Read the model definition and answer for the solid it produces. Units are mm, in the model's axes. Coordinates: 2 decimals unless noted, no trailing zeros. Order: outer loops, then holes, each group sorted by start corner. A loop starts at its lowest first (then second) coordinate and runs counter-clockwise, first axis right, second up. Notation, with made-up numbers: (24, 71.25) - (55, 71.25) arc R15 cw to (55, 80.25) - close; hole circle Ø10 at (-10.5, -17.75). An arc over 180 degrees is marked (long way). Use one line per item in the form item = value.
Autodesk Inventor part; units mm, degrees
ref_plane "YZ Plane" through (0, 0, 0) normal (1, 0, 0) x (0, 1, 0)
ref_plane "XZ Plane" through (0, 0, 0) normal (0, 1, 0) x (-1, 0, 0)
ref_plane "XY Plane" through (0, 0, 0) normal (0, 0, 1) x (1, 0, 0)
sketch "Sketch1" plane through (0, 0, 0) normal (0, 0, 1) x (1, 0, 0)
  line L0 (583, 0) -> (583, -566)
  line L1 (613.4835, 107.0681) -> (1060.6433, 107.0681)
  point P0 (0, 0)
sketch "Sketch2" plane through (0, 0, 0) normal (0, 0, 1) x (1, 0, 0)
  line L0 (583, 0) -> (613.4835, 107.0681)
  line L1 (613.4835, 107.0681) -> (673.4835, 107.0681)
  line L2 (583, 0) -> (583, -105)
  line L3 (673.4835, 105.4681) -> (614.6916, 105.4681)
  line L4 (614.6916, 105.4681) -> (584.6, -0.2233)
  line L5 (584.6, -0.2233) -> (584.6, -105)
  line L6 (583, -105) -> (584.6, -105)
  line L7 (673.4835, 107.0681) -> (673.4835, 105.4681)
  point P0 (0, 0)
  dimension "d0" = 105
  dimension "d1" = 60
  dimension "d2" = 1.6
extrude "Extrusion1" add sketch "Sketch2" against normal blind 1200
sketch "Sketch3" plane through (583, -105, -1200) normal (0, -1, 0) x (1, 0, 0)
  point P0 (-583, 1200)
properties part number "front" material "Steel"
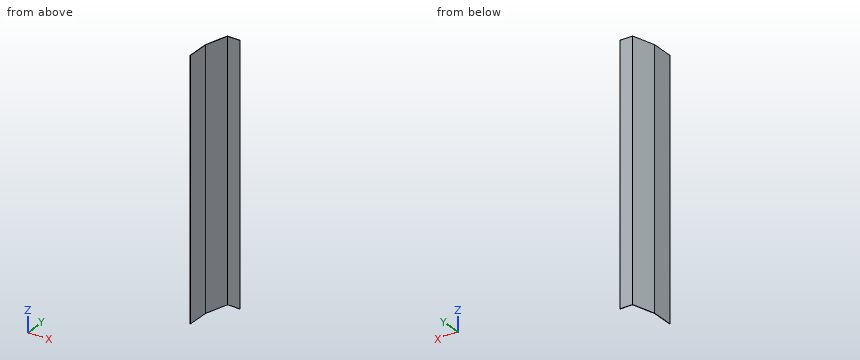
(1) Section A-A, the plane z = -770 is taken. Write down the section's boundary in (x, y).
Answer list:
outline = (583, -105) - (584.6, -105) - (584.6, -0.22) - (614.69, 105.47) - (673.48, 105.47) - (673.48, 107.07) - (613.48, 107.07) - (583, 0) - close
(2) Section B-B, the plane y = -53.5 is taken. Write down the section's boundary in (x, z).
Answer list:
outline = (583, -1200) - (584.6, -1200) - (584.6, 0) - (583, 0) - close
(3) Section C-C, the plane x = 654.5 is taken. Write down the section's boundary in (y, z), then the cut area to 3 significant figures.
Answer list:
outline = (105.47, -1200) - (107.07, -1200) - (107.07, 0) - (105.47, 0) - close
area = 1,920 mm2
(4) Straight lines are drawn through the part: L1, parallel to Y at x = 652.5, z = -270; L2, parallel to X at y = -7.5, z = -239.5; L3, parallel to X at y = 33, z = -437. For each, find the intervals that lie inside material, in ascending order.
Answer list:
L1 = 105.47 to 107.07
L2 = 583 to 584.6
L3 = 592.4 to 594.06
(5) Given pin 1 Ø1 at (x, z) = (651, -803) entering from -Y; pin 2 Ø3 at (y, z) = (32.5, -201.5) entering from -X; pin 3 Ø10 at (y, z) = (74.5, -339.5) entering from -X, each flat-ended and moving along its own axis, determine where each tip first touches the part or whether it passes through.
Answer list:
pin_1 = 105.47
pin_2 = 591.83
pin_3 = 602.79
